from build123d import *

# Parameters (mm, degrees)
F1_DEPTH = 10


with BuildPart() as f1:
    # F0 (on Front) → F1 (new body)
    with BuildSketch(Plane.XZ):
        Polygon((-979.948978, 439.999997), (-980, 0), (-670, 0), (-670, 443.162907), align=None)
        Polygon((-670, 443.162907), (-670, 0), (-310, 0), (-310, 446.836569), align=None)
        Polygon((-310, 446.836569), (-310, 0), (0, 0), (0, 450), align=None)
    extrude(amount=F1_DEPTH)


solid = f1.part
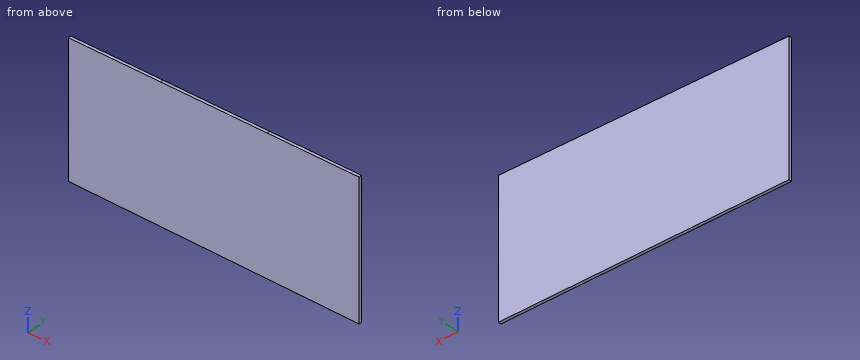
Geometry: final body of the model. Coordinates: model frame, mm. Give positions to 0.01 mm unless a question says otherwise; leave off trailing zeros. Write each loop counter-clockwise with the first axis right and the second up, starting at its lowest first coordinate (ties: lowest second). Pieces come first, ordered by that corner, then holes.
(1) Cut plane B-B, the plane x = -839. Return loops of the section in (y, z).
(2) Ray query, line 1 (X direction, y = -4.25, z = 84); line 2 (Z direction, x = -831, y = -1.25); line 3 (Z direction, x = -567.5, y = -2). Return the intervals inside material, ascending.
(3) First-contact query: P1, Ø5, axis at y = -8.5, z = 110.5, coming from the -X side. Flat tip, straight axial feed; report the tip coordinate or a pass-through.
(4) Cut plane A-A, the plane x = -696. Return loops of the section in (y, z).
Values follow:
1. outline: (-10, 0) - (0, 0) - (0, 441.44) - (-10, 441.44) - close
2. line 1: x = -979.99 to 0
2. line 2: z = 0 to 441.52
2. line 3: z = 0 to 444.21
3. P1: stops at x = -979.99
4. outline: (-10, 0) - (0, 0) - (0, 442.9) - (-10, 442.9) - close
